For this review, take the finished solid that the model builds, in its own axes (mm). Round coordinates to 2 decimals unless told otherwise and drop trailing zeros. Order: outer loops, then holes, each group sorted by start corner. A loop starts at its lowest first (then second) coordinate and runs counter-clockwise, first axis right, second up. Notation, with made-up numbers: (58.25, 46) - (105.25, 46) arc R20 ccw to (105.25, 60) - close; hole circle Ø8 at (-5.75, 38). An arc over 180 degrees is marked (long way). One line per item, written item: value.
```python
from build123d import *

# Parameters (mm, degrees)
SKETCH1_R            = 1.5
BOSS_EXTRUDE1_DEPTH  = 3
M3_CLEARANCE_HOLE1_D = 3.6
CUT_EXTRUDE1_DEPTH   = 10


with BuildPart() as part:
    # Sketch1 → Boss-Extrude1 (new body)
    with BuildSketch(Plane(origin=(0, 0, 0), x_dir=(0, 0, -1), z_dir=(1, 0, 0))):
        with BuildLine():
            Line((33, 103.968745116), (33, 127.468745116))
            ThreePointArc((33, 127.468745116), (32.121320344, 129.590065459), (30, 130.468745116))
            Line((30, 130.468745116), (26.5, 130.468745116))
            ThreePointArc((26.5, 130.468745116), (7.761670299, 122.707074817), (0, 103.968745116))
            Line((0, 103.968745116), (0, 0))
            Line((0, 0), (33, 0))
            Line((33, 0), (33, 103.968745116))
        make_face()
        with Locations((4, 4)):
            Circle(SKETCH1_R, mode=Mode.SUBTRACT)
        with Locations((29, 4)):
            Circle(SKETCH1_R, mode=Mode.SUBTRACT)
        with Locations((26.5, 103.968745116)):
            Circle(SKETCH1_R, mode=Mode.SUBTRACT)
        with BuildLine():
            ThreePointArc((4.7, 103.968745116), (11.08507217, 119.383672946), (26.5, 125.768745116))
            ThreePointArc((26.5, 125.768745116), (28.3, 123.968745116), (26.5, 122.168745116))
            ThreePointArc((26.5, 122.168745116), (13.630656582, 116.838088533), (8.3, 103.968745116))
            ThreePointArc((8.3, 103.968745116), (6.5, 102.168745116), (4.7, 103.968745116))
        make_face(mode=Mode.SUBTRACT)
    extrude(amount=BOSS_EXTRUDE1_DEPTH)

    # M3 Clearance Hole1 (through all)
    with Locations(Plane.ZY):
        with Locations((-29, 4), (-4, 4), (-26.5, 103.968745116)):
            Hole(M3_CLEARANCE_HOLE1_D / 2)

    # Sketch4 → Cut-Extrude1 (cut)
    with BuildSketch(Plane(origin=(3, 0, 0), x_dir=(0, 0, -1), z_dir=(1, 0, 0))):
        Polygon((5, 13.619501596), (13.039872779, 22.021779252), (5, 30.424056909), align=None)
        Polygon((7.5, 9), (25.5, 9), (16.5, 18.405683521), align=None)
        Polygon((28, 30.424056909), (19.960127221, 22.021779252), (28, 13.619501596), align=None)
        Polygon((5, 37.656248372), (16.5, 25.637874984), (28, 37.656248372), (28, 39.656248372), (16.5, 50.541969576), (5, 39.656248372), align=None)
        Polygon((20.136657006, 53.984372558), (28, 46.541054335), (28, 61.427690781), align=None)
        Polygon((5, 61.427690781), (5, 46.541054335), (12.863342994, 53.984372558), align=None)
        Polygon((5, 70.312496744), (5, 68.312496744), (16.5, 57.426775539), (28, 68.312496744), (28, 70.312496744), (16.5, 82.330870131), align=None)
        Polygon((19.960127221, 85.946965863), (28, 77.544688207), (28, 94.349243519), align=None)
        Polygon((5, 94.349243519), (5, 77.544688207), (13.039872779, 85.946965863), align=None)
        Polygon((7.5, 98.968745116), (16.5, 89.563061595), (25.5, 98.968745116), align=None)
    extrude(amount=-CUT_EXTRUDE1_DEPTH, mode=Mode.SUBTRACT)


solid = part.part
```
Item 1: Take a section at D-D (y = 4). Write out the cut boundary in (x, z), plus the area to 3 significant figures.
Returned:
outline: (0, -33) - (3, -33) - (3, -30.8) - (0, -30.8) - close; (0, -27.2) - (3, -27.2) - (3, -5.8) - (0, -5.8) - close; (0, -2.2) - (3, -2.2) - (3, 0) - (0, 0) - close
area: 77.4 mm^2
Item 2: For P1, Ø1.5, axis at x = 1.5, z = -16.5, coming from the +Y side, flat-tipped, find the tip position at first contact; note if it passes through.
Returned:
P1: y = 128.8
Item 3: Wall thickness on line 1 (Y direction, x = 0.75, z = -29); line 2 (Z direction, x = 2.45, y = 103.5); line 3 (Z direction, x = 0.65, y = 58): over which ranges is each line inside the solid? List them lowest first.
Returned:
line 1: 0 to 2.2, 5.8 to 130.47
line 2: -33 to -28.24, -24.76 to -8.24, -4.76 to 0
line 3: -33 to -28, -24.38 to -17.11, -15.89 to -8.62, -5 to 0
Item 4: The part is to be moulded in two halves that separate along Y. For faces 1 (the flat face through (0, 66, -27)), 2 (the cylindrical face through (1.48, 129.57, -32.14)), 3 (the flat face through (2, 86, -5)), say which applies: +Y half, -Y half, draft (parallel to the pull), parting line (faces both ways), or undercut.
Returned:
face 1: draft
face 2: +Y half
face 3: undercut
Item 5: Take a section at A-A (y = 84). Write out the cut boundary in (x, z), plus the area to 3 significant figures.
Returned:
outline: (0, -33) - (3, -33) - (3, -28) - (0, -28) - close; (0, -21.82) - (3, -21.82) - (3, -11.18) - (0, -11.18) - close; (0, -5) - (3, -5) - (3, 0) - (0, 0) - close
area: 61.9 mm^2
Item 6: Take a section at B-B (y = 63.5). Write out the cut boundary in (x, z).
Returned:
outline: (0, -33) - (3, -33) - (3, -22.92) - (0, -22.92) - close; (0, -10.08) - (3, -10.08) - (3, 0) - (0, 0) - close
Item 7: Take a section at C-C (x = 2.1). Count the separate pieces of the cut face and the enclosed holes in it, plus the area to 3 significant figures.
Returned:
separate pieces: 1
enclosed holes: 14
area: 2,820 mm^2
